Autodesk Inventor part; units mm, degrees
ref_plane "YZ Plane" through (0, 0, 0) normal (1, 0, 0) x (0, 1, 0)
ref_plane "XZ Plane" through (0, 0, 0) normal (0, 1, 0) x (-1, 0, 0)
ref_plane "XY Plane" through (0, 0, 0) normal (0, 0, 1) x (1, 0, 0)
sketch "Sketch1" plane through (0, 0, 0) normal (0, 1, 0) x (-1, 0, 0)
  line L0 (32.5, -9.5) -> (-32.5, -9.5)
  line L1 (-32.5, -9.5) -> (-32.5, 9.5)
  line L2 (-32.5, 9.5) -> (32.5, 9.5)
  line L3 (32.5, 9.5) -> (32.5, -9.5)
  point P0 (0, 0)
  point P1 (0, -9.5)
  point P2 (32.5, 0)
  dimension "d0" = 65
  dimension "d1" = 19
extrude "Extrusion1" add sketch "Sketch1" along normal blind 16
sketch "Sketch2" plane through (0, 16, 0) normal (0, 1, 0) x (1, 0, 0)
  line L0 (-28.25, 6) -> (-5.25, 6)
  line L1 (-5.25, 6) -> (-5.25, -6)
  line L2 (-5.25, -6) -> (-28.25, -6)
  line L3 (-28.25, -6) -> (-28.25, 6)
  line L4 (0, 13.3) -> (0, -13.3) construction
  line L5 (-32.5, 9.5) -> (-32.5, -9.5)
  line L6 (28.25, 6) -> (5.25, 6)
  line L7 (5.25, 6) -> (5.25, -6)
  line L8 (5.25, -6) -> (28.25, -6)
  line L9 (28.25, -6) -> (28.25, 6)
  point P0 (0, 0)
  point P1 (-5.25, 0)
  dimension "d4" = 23
  dimension "d5" = 12
  dimension "d9" = 4.25
extrude "Extrusion2" cut sketch "Sketch2" against normal through all
chamfer "Chamfer1" distance 2.5 angle 45 4 edges at (-32.5, 8, 9.5) (-32.5, 8, -9.5) (32.5, 8, 9.5) (32.5, 8, -9.5)
chamfer "Chamfer2" distance 2 angle 45 4 edges at (0, 16, -9.5) (0, 16, 9.5) (0, 0, 9.5) (0, 0, -9.5)
sketch "Sketch3" plane through (-30, 2, 9.5) normal (0, 0, 1) x (1, 0, 0)
  line L0 (-2.5, 8.5) -> (62.5, 8.5)
  line L1 (62.5, 8.5) -> (62.5, 3.5)
  line L2 (62.5, 3.5) -> (-2.5, 3.5)
  line L3 (-2.5, 3.5) -> (-2.5, 8.5)
  line L4 (-2.5, 14) -> (-2.5, -2)
  line L5 (62.5, -2) -> (62.5, 14)
  point P0 (30, -2)
  point P1 (62.5, 6)
  point P2 (62.5, 6)
  dimension "d18" = 5
extrude "Extrusion3" cut sketch "Sketch3" against normal blind 2
sketch "Sketch5" plane through (30, 2, -9.5) normal (0, 0, -1) x (-1, 0, 0)
  line L0 (-2.5, 3.5) -> (62.5, 3.5)
  line L1 (62.5, 3.5) -> (62.5, 8.5)
  line L2 (62.5, 8.5) -> (-2.5, 8.5)
  line L3 (-2.5, 8.5) -> (-2.5, 3.5)
  line L4 (-2.5, 14) -> (-2.5, -2)
  line L5 (62.5, -2) -> (62.5, 14)
  point P0 (30, -2)
  point P1 (62.5, 6)
  point P2 (62.5, 6)
  dimension "d21" = 5
extrude "Extrusion4" cut sketch "Sketch5" against normal blind 2
sketch "Sketch6" plane through (-32.5, 0, -7) normal (-1, 0, 0) x (0, 0, 1)
  line L0 (-0.5, 5.5) -> (-2.5, 5.5)
  line L1 (16.5, 10.5) -> (-2.5, 10.5)
  line L2 (-2.5, 10.5) -> (-2.5, 5.5)
  line L3 (-2.5, 5.5) -> (16.5, 5.5)
  line L4 (16.5, 5.5) -> (16.5, 10.5)
  point P0 (7, 0)
  point P1 (16.5, 5.5)
  point P2 (-2.5, 10.5)
extrude "Extrusion5" cut sketch "Sketch6" against normal blind 2
sketch "Sketch7" plane through (32.5, 0, 7) normal (1, 0, 0) x (0, 0, -1)
  line L0 (0, 10.5) -> (-2.5, 10.5)
  line L1 (-2.5, 10.5) -> (16.5, 10.5)
  line L2 (16.5, 10.5) -> (16.5, 5.5)
  line L3 (16.5, 5.5) -> (-2.5, 5.5)
  line L4 (-2.5, 5.5) -> (-2.5, 10.5)
  point P0 (7, 0)
extrude "Extrusion6" cut sketch "Sketch7" against normal blind 2
sketch "Sketch8" plane through (32.5, 16, 7) normal (1, 0, 0) x (0, 0, -1)
  line L0 (4.825, -3.95) -> (9.175, -3.95)
  line L1 (9.175, -3.95) -> (9.175, -5.5)
  line L2 (9.175, -5.5) -> (4.825, -5.5)
  line L3 (4.825, -5.5) -> (4.825, -3.95)
  line L4 (4.825, -10.5) -> (9.175, -10.5)
  line L5 (9.175, -10.5) -> (9.175, -12.05)
  line L6 (9.175, -12.05) -> (4.825, -12.05)
  line L7 (4.825, -12.05) -> (4.825, -10.5)
  line L8 (14, -16) -> (0, -16)
  line L9 (0, -5.5) -> (14, -5.5)
  line L10 (14, -10.5) -> (0, -10.5)
  point P0 (7, -16)
  point P1 (7, -3.95)
  point P2 (7, -10.5)
  point P3 (7, -12.05)
  point P4 (7, -16)
  dimension "d28" = 4.35
  dimension "d29" = 1.55
extrude "Extrusion7" cut sketch "Sketch8" against normal through all
sketch "Sketch9" plane through (0, 16, 0) normal (0, 1, 0) x (1, 0, 0)
  circle A0 centre (30.75, 0) radius 1
  circle A1 centre (2.75, 0) radius 1
  line L0 (0, 13.3) -> (0, -13.3)
  line L1 (28.25, 6) -> (28.25, -6)
  line L2 (5.25, -6) -> (5.25, 6)
  circle A2 centre (-30.75, 0) radius 1
  circle A3 centre (-2.75, 0) radius 1
  point P0 (0, 0)
  dimension "d32" = 2
  dimension "d33" = 1.5
  dimension "d34" = 1.5
extrude "Extrusion8" cut sketch "Sketch9" against normal up to surface (3.95 mm away)
sketch "Sketch10" plane through (0, 0, 0) normal (0, -1, 0) x (1, 0, 0)
  line L0 (0, -13.3) -> (0, 13.3)
  circle A0 centre (-30.75, 0) radius 1
  circle A1 centre (-2.75, 0) radius 1
  line L1 (-28.25, -6) -> (-28.25, 6)
  line L2 (-5.25, 6) -> (-5.25, -6)
  circle A2 centre (30.75, 0) radius 1
  circle A3 centre (2.75, 0) radius 1
  point P0 (0, 0)
  dimension "d37" = 2
  dimension "d38" = 1.5
  dimension "d39" = 1.5
extrude "Extrusion9" cut sketch "Sketch10" against normal up to surface (3.95 mm away)
equation "\"d4\" = servo_A"
equation "\"d5\" = servo_B"
equation "\"d9\" = -0.5 * servo_A + 0.5 * servo_D"
equation "\"d18\" = servo_K"
equation "\"d21\" = servo_K"
equation "\"d28\" = nut_A"
equation "\"d29\" = nut_B"
equation "\"d32\" = servo_H"
equation "\"d33\" = servo_L"
equation "\"d34\" = servo_L"
equation "\"d37\" = servo_H"
equation "\"d38\" = servo_L"
equation "\"d39\" = servo_L"
properties part number "FEMUR2_A"
Here's how the part is built. I have some questions about the finished solid (model axes, mm). A direction names the side the tool comes from. Give positions to 0.01 mm unless a question says otherwise; leave off trailing zeros. Order: outer loops, then holes, each group sorted by start corner. A loop starts at its lowest first (then second) coordinate and runs counter-clockwise, first axis right, second up. Notation, with made-up numbers: (80.25, 43) -> (115.25, 43) arc R34 cw to (115.25, 79) -> close; hole circle Ø9 at (83, 45.5). An arc over 180 degrees is marked (long way). One line per item, written item: value. Start each with the question number.
1. Imagine slicing it at C-C, the plane x = -15. List the corners of the cut face in (y, z) for me, plus the area to 3 significant figures.
2. We'd pull the mould along X, two halves only. Please class faces 1 (the face through (1.96, 14.05, 0.61)), 2 (the face through (0, 5.5, -8)), 3 (the face through (-17, 8, -6)), 4 (the face through (32.5, 13, 0)): released by +X, released by -X, zero draft, split by the parting line, or undercut.
3. I need wall thicknesses on probe 1 along X at (y, z) = (12.75, -3.5); probe 2 along X at (y, z) = (9, 5.75); probe 3 along Y at (x, z) = (-2, 0.75). Which ranges of each line are inside material? Lowest first, please. Write a range as from..to.
4. Imagine slicing it at D-D, the plane y = 1.25. List the corners of the cut face in (x, z) for me, plus the area to 3 significant figures.
5. For faces 5 (the face through (-28.25, 8, 0)), 6 (the face through (0, 4, 9.5)), 7 (the face through (30.5, 8, 0)), 8 (the face through (-3.54, 14.05, 0.61)), 9 (the face through (-30, 11, 2.175)), which set-ups out of +Z, -Z, +X, -X, +Y, -Y let a thin tool reach every point of the face, with its end or its side?
6. Imagine slicing it at A-A, the plane z = 4.5. List the corners of the cut face in (x, y) for me.
7. Will these pins go through, and if not, where does the flat tip stop? pin 1 Ø2.5 at (x, z) = (-30.75, 0) entering from +Y; pin 2 Ø1.5 at (x, y) = (-10.5, 9.5) entering from +Z; pin 3 Ø1.6 at (x, z) = (-30.75, 0) entering from -Y.
8. Imagine slicing it at B-B, the plane y = 9. List the corners of the cut face in (x, z) for me, plus the area to 3 significant figures.
Values follow:
1. outline: (0, -7.5) -> (2, -9.5) -> (5.5, -9.5) -> (5.5, -7.5) -> (10.5, -7.5) -> (10.5, -9.5) -> (14, -9.5) -> (16, -7.5) -> (16, -6) -> (0, -6) -> close; (0, 6) -> (16, 6) -> (16, 7.5) -> (14, 9.5) -> (10.5, 9.5) -> (10.5, 7.5) -> (5.5, 7.5) -> (5.5, 9.5) -> (2, 9.5) -> (0, 7.5) -> close
1. area: 84.0 mm2
2. face 1: undercut
2. face 2: zero draft
2. face 3: undercut
2. face 4: released by +X
3. probe 1: x = -32.5..-28.25, -5.25..5.25, 28.25..32.5
3. probe 2: x = -30.5..-28.25, -5.25..5.25, 28.25..30.5
3. probe 3: y = 0..3.95, 5.5..10.5, 12.05..16
4. outline: (-32.5, -7) -> (-30.75, -8.75) -> (30.75, -8.75) -> (32.5, -7) -> (32.5, 7) -> (30.75, 8.75) -> (-30.75, 8.75) -> (-32.5, 7) -> close; hole circle Ø2 at (-30.75, 0); hole (-28.25, -6) -> (-5.25, -6) -> (-5.25, 6) -> (-28.25, 6) -> close; hole circle Ø2 at (-2.75, 0); hole circle Ø2 at (2.75, 0); hole (5.25, -6) -> (28.25, -6) -> (28.25, 6) -> (5.25, 6) -> close; hole circle Ø2 at (30.75, 0)
4. area: 567 mm2
5. face 5: +Y, -Y
5. face 6: +Z, +X, -X, +Y, -Y
5. face 7: +Z, -Z, +X
5. face 8: +Y
5. face 9: +X, -X
6. outline: (-32.5, 0) -> (-28.25, 0) -> (-28.25, 16) -> (-32.5, 16) -> (-32.5, 10.5) -> (-30.5, 10.5) -> (-30.5, 5.5) -> (-32.5, 5.5) -> close; (-5.25, 0) -> (5.25, 0) -> (5.25, 16) -> (-5.25, 16) -> close; (28.25, 0) -> (32.5, 0) -> (32.5, 5.5) -> (30.5, 5.5) -> (30.5, 10.5) -> (32.5, 10.5) -> (32.5, 16) -> (28.25, 16) -> close
7. pin 1: stops at y = 16
7. pin 2: stops at z = 7.5
7. pin 3: stops at y = 5.5
8. outline: (-30.5, -7.5) -> (30.5, -7.5) -> (30.5, 7.5) -> (-30.5, 7.5) -> close; hole (-28.25, -6) -> (-5.25, -6) -> (-5.25, 6) -> (-28.25, 6) -> close; hole (5.25, -6) -> (28.25, -6) -> (28.25, 6) -> (5.25, 6) -> close
8. area: 363 mm2
